from build123d import *

# Parameters (mm, degrees)
F1_DEPTH = 25
F2_R     = 5.5
F2_R_2   = 4.5
F3_DEPTH = 5
F4_DEPTH = 5
F5_R     = 4.5
F6_DEPTH = 5


# Not quite as in the source:
# - ends of sketch curves that miss each other by under 0.0002 mm in the source are joined


with BuildPart() as f1:
    # F0 (on Front) → F1 (new body)
    with BuildSketch(Plane.XZ):
        with BuildLine():
            Line((134, 0), (134, 5))
            Line((134, 5), (5, 5))
            ThreePointArc((5, 5), (2.4118095455, 4.6592580848), (0, 3.6602538402))
            Line((0, 3.6602538402), (0, 0))
            Line((0, 0), (5, 0))
            Line((5, 0), (134, 0))
        make_face()
        with BuildLine():
            Line((0, 0), (0, 3.6602538402))
            ThreePointArc((0, 3.6602538402), (-3.6602539143, -1.284e-07), (-4.9999998289, -5))
            Line((-4.9999998289, -5), (-5, -76))
            Line((-5, -76), (0, -76))
            Line((0, -76), (0, -5))
            Line((0, -5), (0, 0))
        make_face()
        with BuildLine():
            ThreePointArc((0, -5), (1.4644660941, -1.4644660941), (5, 0))
            Line((5, 0), (0, 0))
            Line((0, 0), (0, -5))
        make_face()
    extrude(amount=-F1_DEPTH)

    # F2 (on face) → F3 (cut)
    with BuildSketch(Plane.XY.offset(5)):
        with Locations((114, 12.5)):
            Circle(F2_R)
        with Locations((84, 12.5)):
            Circle(F2_R_2)
        with Locations((45, 12.5)):
            Circle(F2_R_2)
    extrude(amount=-F3_DEPTH, mode=Mode.SUBTRACT)

    # F2 (on face) → F4 (cut)
    with BuildSketch(Plane.XY.offset(5)):
        with Locations((114, 12.5)):
            Circle(F2_R)
        with Locations((84, 12.5)):
            Circle(F2_R_2)
        with Locations((45, 12.5)):
            Circle(F2_R_2)
    extrude(amount=-F4_DEPTH, mode=Mode.SUBTRACT)

    # F5 (on face) → F6 (cut)
    with BuildSketch(Plane(origin=(-5, 0, 0), x_dir=(0, -1, 0), z_dir=(-1, 0, 0))):
        with Locations((-12.5, -66)):
            Circle(F5_R)
    extrude(amount=-F6_DEPTH, mode=Mode.SUBTRACT)


solid = f1.part
Could you check a few things on this model? Use its own coordinates, in mm. A direction names the side the tool comes from. Give positions to 0.01 mm unless a question says otherwise; leave off trailing zeros. Order: outer loops, then holes, each group sorted by start corner. A loop starts at its lowest first (then second) coordinate and runs counter-clockwise, first axis right, second up. Notation, with made-up numbers: (41, 63.5) -> (96, 63.5) arc R7 cw to (96, 76.5) -> close; hole circle Ø2 at (74, 67.5). An arc over 180 degrees is marked (long way). Answer in a Markdown table with one row per item. Add a question column.
Item 1: For faces 4 (the flat face through (0, 12, -41)), 5 (the flat face through (70, 12, 5)), which set-ups out of +Z, -Z, +X, -X, +Y, -Y let a thin tool reach every point of the face, with its end or its side?
Item 2: I'm going to push flat-ended pins straight in: P1, Ø1, axis at x = 86.5, y = 3, coming from the -Z side; P2, Ø7, axis at x = 84, y = 12.5, coming from the -Z side; P3, Ø1, axis at y = 17.5, z = -50, coming from the +X side. Where does each tip first touch, or does it pass through?
Item 3: We'd pull the mould along X, two halves only. Please class faces 1 (the cylindrical face through (79.504, 12.698, 2.535)), 2 (the cylindrical face through (1, 12, -2)), 3 (the flat face through (-3, 12, -76)): pulls with the +X half, pulls with the -X half, needs draft (parallel to the pull), parting line crosses it, or undercut.
Item 4: Please list where these lines run through material, in increasing order: probe 1 along Y at (x, z) = (84, 2.8); probe 2 along X at (y, z) = (4, -39.5); probe 3 along Z at (x, y) = (-1.15, 12.5).
Item 5: Imagine slicing it at D-D (y = 23). List the corners of the cut face in (x, z) for me, and give its area (3 significant figures).
Item 6: Imagine slicing it at C-C (y = 12.5). List the corners of the cut face in (x, z) for me.
Item 7: Imagine slicing it at B-B (x = 45). List the corners of the cut face in (y, z) for me.
Item 8: Imagine slicing it at A-A (z = -66). List the corners of the cut face in (x, y) for me.
Result:
| question | item | result |
|---|---|---|
| 1 | face 4 | -Z, +X, +Y, -Y |
| 1 | face 5 | +Z, +X, -X, +Y, -Y |
| 2 | P1 | z = 0 |
| 2 | P2 | through |
| 2 | P3 | x = 0 |
| 3 | face 1 | undercut |
| 3 | face 2 | pulls with the +X half |
| 3 | face 3 | needs draft |
| 4 | probe 1 | 0 to 8, 17 to 25 |
| 4 | probe 2 | -5 to 0 |
| 4 | probe 3 | -76 to -70.5, -61.5 to 2.89 |
| 5 | outline | (-5, -76) -> (0, -76) -> (0, -5) arc R5 cw to (5, 0) -> (134, 0) -> (134, 5) -> (5, 5) arc R10 ccw to (0, 3.66) arc R10 ccw to (-5, -5) -> close |
| 5 | area | 1,060 mm2 |
| 6 | outline | (-5, -76) -> (0, -76) -> (0, -70.5) -> (-5, -70.5) -> close; (-5, -61.5) -> (0, -61.5) -> (0, -5) arc R5 cw to (5, 0) -> (40.5, 0) -> (40.5, 5) -> (5, 5) arc R10 ccw to (0, 3.66) arc R10 ccw to (-5, -5) -> close; (49.5, 0) -> (79.5, 0) -> (79.5, 5) -> (49.5, 5) -> close; (88.5, 0) -> (108.5, 0) -> (108.5, 5) -> (88.5, 5) -> close; (119.5, 0) -> (134, 0) -> (134, 5) -> (119.5, 5) -> close |
| 7 | outline | (0, 0) -> (8, 0) -> (8, 5) -> (0, 5) -> close; (17, 0) -> (25, 0) -> (25, 5) -> (17, 5) -> close |
| 8 | outline | (-5, 0) -> (0, 0) -> (0, 8) -> (-5, 8) -> close; (-5, 17) -> (0, 17) -> (0, 25) -> (-5, 25) -> close |
